Input: dimensioned drawing with shaded views. Units: mm. Origin: part minimum x, y, z. Round coordinates to 2 decimals unless told otherwise and drop trailing zeros. Loops run counter-clockwise (first coordinate to the right, second up) from the corner with the lowest first, then second, coordinate; pieces in that order, holes last. Notation, with made-up numbers: (-39, -34.5) - (-16, -34.5) arc R11 ccw to (-16, -30.5) - close; hole circle Ø10 at (32, 50). An arc over 180 degrees is marked (long way). One line per question, with ' | ' between items.
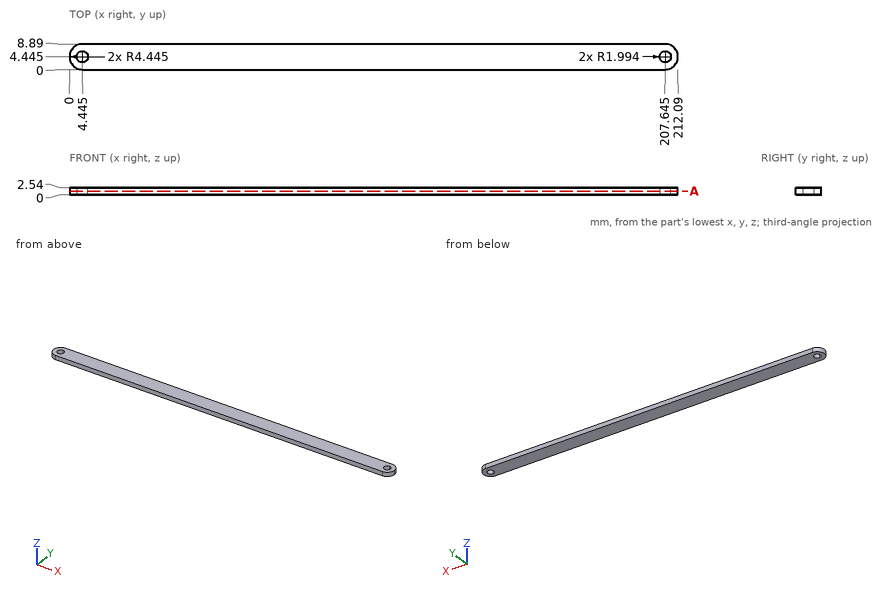
1. Material intervals for probe 1 along X at (y, z) = (4, 0.85); probe 2 along X at (y, z) = (3.25, 0.6); probe 3 along X at (y, z) = (8, 0.95), sorted ascending.
Worked out:
probe 1: x = 0.02 to 2.5, 6.39 to 205.7, 209.59 to 212.07 | probe 2: x = 0.16 to 2.85, 6.04 to 206.05, 209.24 to 211.93 | probe 3: x = 1.78 to 210.31
2. Section query A-A, the plane z = 1.3. Return loops of the section in (x, y) (3 decimals).
Worked out:
outline: (4.445, 0) - (207.645, 0) arc R4.445 ccw to (207.645, 8.89) - (4.445, 8.89) arc R4.445 ccw to start; hole circle Ø3.988 at (4.445, 4.445); hole circle Ø3.988 at (207.645, 4.445)
3. Contact query for a flat-ended pin moving along its axis: P1, Ø1, axis at y = 1.5, z = 1.5, coming from the +X side. Output: stop coordinate, or through.
Worked out:
P1: stops at x = 211.36
